from build123d import *

# Parameters (mm, degrees)
F1_DEPTH      = 101.6
F3_DEPTH      = 25.4
F3_DEPTH_BACK = 25.4
F4_R          = 6.35
F5_R          = 5.159375
F6_DEPTH      = 25.4
F6_DEPTH_BACK = 25.4


with BuildPart() as f1:
    # F0 (on Front) → F1 (new body, symmetric)
    with BuildSketch(Plane.XZ):
        with BuildLine():
            Line((-2.921, 88.9), (-25.93848, 88.9))
            Line((-25.93848, 88.9), (-25.93848, 85.471))
            Line((-25.93848, 85.471), (-3.175, 85.471))
            ThreePointArc((-3.175, 85.471), (-0.9299359697, 84.5410640303), (0, 82.296))
            Line((0, 82.296), (0, 0))
            Line((0, 0), (3.429, 0))
            Line((3.429, 0), (3.429, 82.55))
            ThreePointArc((3.429, 82.55), (1.5691280605, 87.0401280605), (-2.921, 88.9))
        make_face()
    extrude(amount=F1_DEPTH, both=True)

    # F2 (on face) → F3 (cut, two sides)
    with BuildSketch(Plane.YZ.offset(3.429)) as f3_sk:
        Polygon((-53.975, 0), (-101.6, 47.625), (-101.6, 0), align=None)
        Polygon((101.6, 0), (101.6, 47.625), (53.975, 0), align=None)
    extrude(amount=-F3_DEPTH, mode=Mode.SUBTRACT)
    extrude(f3_sk.sketch, amount=F3_DEPTH_BACK, mode=Mode.SUBTRACT)

    # F4
    f4_edges = [f1.edges().sort_by_distance(p)[0] for p in [
        (1.7145, -101.6, 47.625),
        (-25.93848, -101.6, 87.1855),
        (1.7145, -53.975, 0),
        (1.7145, 53.975, 0),
        (1.7145, 101.6, 47.625),
        (-25.93848, 101.6, 87.1855),
    ]]
    fillet(f4_edges, radius=F4_R)

    # F5 (on face) → F6 (cut, two sides)
    with BuildSketch(Plane.YZ.offset(3.429)) as f6_sk:
        with Locations((0, 45.24375)):
            Circle(F5_R)
        with Locations((0, 13.49375)):
            Circle(F5_R)
    extrude(amount=-F6_DEPTH, mode=Mode.SUBTRACT)
    extrude(f6_sk.sketch, amount=F6_DEPTH_BACK, mode=Mode.SUBTRACT)


solid = f1.part
Geometry: final body of the model. Coordinates: model frame, mm. A direction names the side the tool comes from. Give positions to 0.01 mm unless a question says otherwise; leave off trailing zeros. Order: outer loops, then holes, each group sorted by start corner. A loop starts at its lowest first (then second) coordinate and runs counter-clockwise, first axis right, second up. Notation, with made-up numbers: (56.5, 85) -> (84.5, 85) arc R22 ccw to (84.5, 107) -> close; hole circle Ø3 at (61.25, 65.5). An arc over 180 degrees is marked (long way). Write each question's results on one line, items separated by ' | '.
1) Line query: line 1 along Z through (x, y) = (2.75, 0); line 2 along Z through (x, y) = (-6.25, 61); line 3 along X through (y, z) = (47, 20). Output: solid intervals per line, ascending.
Geometry says:
line 1: z = 0 to 8.33, 18.65 to 40.08, 50.4 to 85.41 | line 2: z = 85.47 to 88.9 | line 3: x = 0 to 3.43
2) Draft query along Y for faces 3 (the face through (0.4, -101.6, 75.4)), 4 (the face through (-14, -1, 88.9)), 5 (the face through (1.739, -1.118, 8.457)), 6 (the face through (1.74, -0.67, 50.36)). Return one class per face: released by +Y, released by -Y, zero draft, split by the parting line, or undercut.
Geometry says:
face 3: released by -Y | face 4: zero draft | face 5: undercut | face 6: undercut
3) Cut plane C-C (x = -10.75). Output: boundary loops of the cut face in (y, z).
Geometry says:
outline: (-101.6, 85.47) -> (101.6, 85.47) -> (101.6, 88.9) -> (-101.6, 88.9) -> close
4) Set-up query: faces 1 (the face through (3.429, -1, 32)), 2 (the face through (0, -1, 51)). Return all of +Z, -Z, +X, -X, +Y, -Y with unobstructed straight access to the full face (end or side cutting, diameter ignored); none if empty.
Geometry says:
face 1: +Z, -Z, +X, +Y, -Y | face 2: -Z, -X, +Y, -Y
5) First-contact query: pin 1 Ø12 at (y, z) = (0, 45.24) entering from -X. Flat tip, straight axial feed; report the tip coordinate or a pass-through.
Geometry says:
pin 1: stops at x = 0
6) Cut plane B-B (z = 16). Output: boundary loops of the cut face in (x, y) (3 decimals).
Geometry says:
outline: (0, -69.975) -> (3.429, -69.975) -> (3.429, -4.51) -> (0, -4.51) -> close; (0, 4.51) -> (3.429, 4.51) -> (3.429, 69.975) -> (0, 69.975) -> close
7) Cut plane A-A (y = 0). Output: boundary loops of the cut face in (x, z) (3 decimals), and give its area (3 significant figures).
Geometry says:
outline: (-25.938, 85.471) -> (-3.175, 85.471) arc R3.175 cw to (0, 82.296) -> (0, 50.403) -> (3.429, 50.403) -> (3.429, 82.55) arc R6.35 ccw to (-2.921, 88.9) -> (-25.938, 88.9) -> close; (0, 0) -> (3.429, 0) -> (3.429, 8.334) -> (0, 8.334) -> close; (0, 18.653) -> (3.429, 18.653) -> (3.429, 40.084) -> (0, 40.084) -> close | area: 317 mm²
8) Cut plane D-D (y = 66.5). Output: boundary loops of the cut face in (x, z) (3 decimals).
Geometry says:
outline: (-25.938, 85.471) -> (-3.175, 85.471) arc R3.175 cw to (0, 82.296) -> (0, 12.525) -> (3.429, 12.525) -> (3.429, 82.55) arc R6.35 ccw to (-2.921, 88.9) -> (-25.938, 88.9) -> close
